```python
from build123d import *

# Parameters (mm, degrees)
SKETCH003_W          = 16
SKETCH003_H          = 15
PAD001_DEPTH         = 1.4
THICKNESS_T          = -0.2
SKETCH004_W          = 14.6
SKETCH004_H          = 0.5
POCKET002_DEPTH      = 8.001
POCKET002_DEPTH_BACK = 8.001


with BuildPart() as part:
    # Sketch003 → Pad001 (new body)
    with BuildSketch(Plane.XY):
        Rectangle(SKETCH003_W, SKETCH003_H)
    extrude(amount=PAD001_DEPTH)

    # Thickness
    thickness_openings = [part.faces().sort_by_distance(p)[0] for p in [
        (0, 0, 0),
    ]]
    offset(amount=THICKNESS_T, openings=thickness_openings)

    # Sketch004 → Pocket002 (cut, two sides)
    with BuildSketch(Plane.YZ) as pocket002_sk:
        with Locations((0, 0.25)):
            Rectangle(SKETCH004_W, SKETCH004_H)
    extrude(amount=-POCKET002_DEPTH, mode=Mode.SUBTRACT)
    extrude(pocket002_sk.sketch, amount=POCKET002_DEPTH_BACK, mode=Mode.SUBTRACT)


with BuildPart() as part_1:
    # Body001 placement: moved
    add(part.part.moved(Location((0, 0, 0.6348))))


solid = part_1.part
```
Source: CAD feature listing. Evaluate the final solid. Frame: model axes, mm. A direction names the side the tool comes from. Give positions to 0.01 mm unless a question says otherwise; leave off trailing zeros. Loops run counter-clockwise (first coordinate to the right, second up) from the corner with the lowest first, then second, coordinate; pieces in that order, holes last. Notation, with made-up numbers: (59.25, -35.75) - (88.25, -35.75) arc R19 cw to (88.25, -18.75) - close; hole circle Ø2 at (65.5, 45.25). An arc over 180 degrees is marked (long way). Use CSV: the item, a comma, the result in double quotes.
1) Cut plane B-B (x = -6.25). Output: boundary loops of the cut face in (y, z).
Worked out:
outline,"(-7.5, 0.63) - (-7.3, 0.63) - (-7.3, 1.83) - (7.3, 1.83) - (7.3, 0.63) - (7.5, 0.63) - (7.5, 2.03) - (-7.5, 2.03) - close"
2) Set-up query: faces 1 (the flat face through (0, -7.3, 1)), 2 (the flat face through (0, 0, 2.035)). Return all of +Z, -Z, +X, -X, +Y, -Y with unobstructed straight access to the full face (end or side cutting, diameter ignored); none if empty.
Worked out:
face 1,"-Z"
face 2,"+Z, +X, -X, +Y, -Y"
3) Cut plane C-C (y = -5.5). Output: boundary loops of the cut face in (x, z), and give its area (3 significant figures).
Worked out:
outline,"(-8, 1.13) - (-7.8, 1.13) - (-7.8, 1.83) - (7.8, 1.83) - (7.8, 1.13) - (8, 1.13) - (8, 2.03) - (-8, 2.03) - close"
area,"3.48 mm^2"
4) Cut plane A-A (z = 0.95). Output: boundary loops of the cut face in (x, y), and give its area (3 significant figures).
Worked out:
outline,"(-8, -7.5) - (8, -7.5) - (8, -7.3) - (-8, -7.3) - close; (-8, 7.3) - (8, 7.3) - (8, 7.5) - (-8, 7.5) - close"
area,"6.40 mm^2"
5) Mould query, pull axis X, two halves, no side actions, for faces 3 (the flat face through (0, -7.5, 1)), 4 (the flat face through (0, 0, 1.835)), 5 (the flat face through (8, -0.1, 1.6)). Classes: +X half, -X half, draft (parallel to the pull), parting line (faces both ways), or undercut.
Worked out:
face 3,"draft"
face 4,"undercut"
face 5,"+X half"
6) Line query: line 1 (X direction, y = 6.25, z = 1.6); line 2 (Y direction, x = 0.5, z = 0.95); line 3 (Z direction, x = -3.5, y = -2). Output: solid intervals per line, ascending.
Worked out:
line 1,"x = -8 to -7.8, 7.8 to 8"
line 2,"y = -7.5 to -7.3, 7.3 to 7.5"
line 3,"z = 1.83 to 2.03"
7) Pin query (flat end, axial travel): P1, Ø2, axis at x = -6, y = 5.5, coming from the -Z side. Return the tip coordinate at first contact, or that it passes through.
Worked out:
P1,"stops at z = 1.83"
